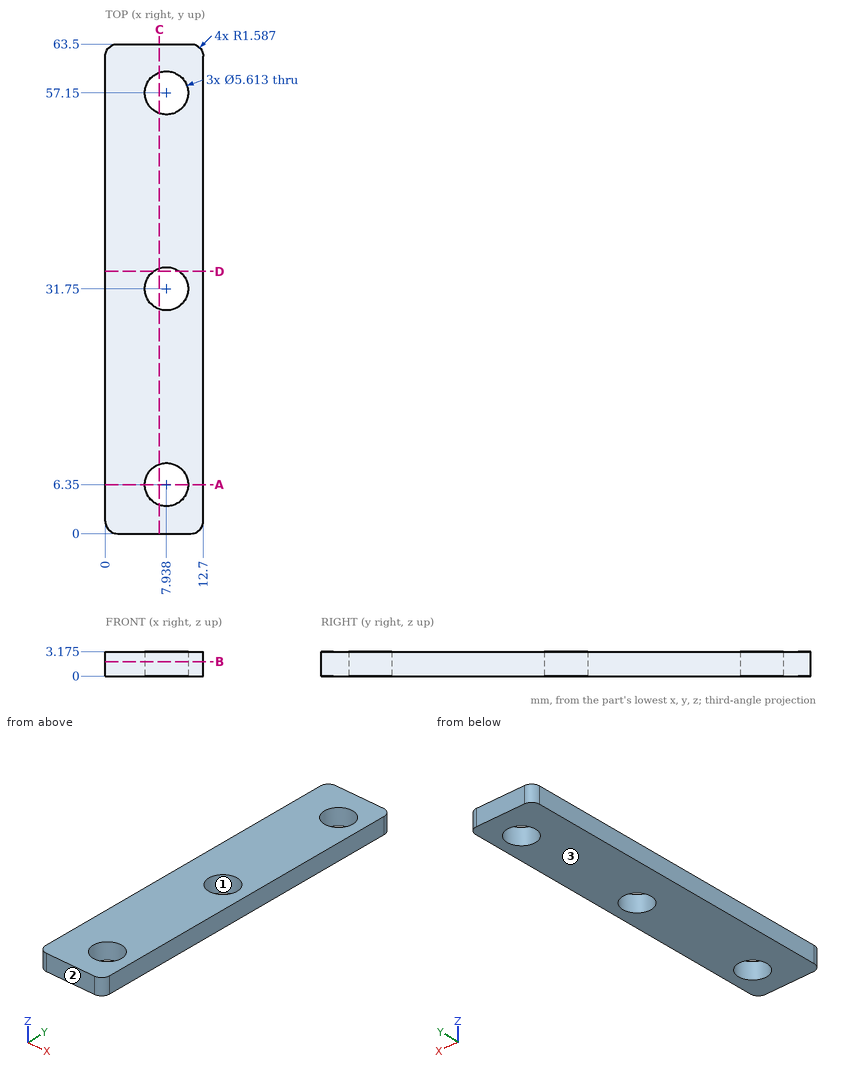
The drawing under review shows one solid part. Ordinate dimensions are in mm from its lowest x, y, z. Round coordinates to 2 decimals unless told otherwise and drop trailing zeros. Order: outer loops, then holes, each group sorted by start corner. A loop starts at its lowest first (then second) coordinate and runs counter-clockwise, first axis right, second up. Notation, with made-up numbers: (88.25, -22.5) - (125.25, -22.5) arc R21 cw to (125.25, -6.5) - close; hole circle Ø4 at (77.5, -4.5). An arc over 180 degrees is marked (long way). Return JSON: item names as keys, results as strings.
Q1. Consider section A-A on y = 6.35. Write out the cut boundary in (x, z) (1 decimal).
Computed values:
{"outline": "(0, 0) - (5.1, 0) - (5.1, 3.2) - (0, 3.2) - close; (10.7, 0) - (12.7, 0) - (12.7, 3.2) - (10.7, 3.2) - close"}
Q2. Consider section C-C on x = 7. Write out the cut boundary in (y, z) (1 decimal), plus the area to 3 significant figures.
Computed values:
{"outline": "(0, 0) - (3.7, 0) - (3.7, 3.2) - (0, 3.2) - close; (9, 0) - (29.1, 0) - (29.1, 3.2) - (9, 3.2) - close; (34.4, 0) - (54.5, 0) - (54.5, 3.2) - (34.4, 3.2) - close; (59.8, 0) - (63.5, 0) - (63.5, 3.2) - (59.8, 3.2) - close", "area": "151 mm2"}
Q3. Consider section B-B on z = 1.85. Give the number of separate pieces and of enclosed holes in the cut face, plus the area to 3 significant figures.
Computed values:
{"separate pieces": "1", "enclosed holes": "3", "area": "730 mm2"}
Q4. Consider section D-D on y = 34. Write out the cut boundary in (x, z) (1 decimal).
Computed values:
{"outline": "(0, 0) - (6.3, 0) - (6.3, 3.2) - (0, 3.2) - close; (9.6, 0) - (12.7, 0) - (12.7, 3.2) - (9.6, 3.2) - close"}
Q5. Wall thickness on L1, parallel to Y at x = 10.5, z = 2.4 (1 decimal); L2, parallel to Y at x = 7.5, z = 0.35; L3, parallel to Y at x = 0.75, z = 2.05: over which ranges is each line inside the solid? List them lowest first. Write a range as [from, to].
Computed values:
{"L1": "y = [0, 5.2], [7.5, 30.6], [32.9, 56], [58.3, 63.5]", "L2": "y = [0, 3.58], [9.12, 28.98], [34.52, 54.38], [59.92, 63.5]", "L3": "y = [0.24, 63.26]"}
Q6. The part is to be moulded in two halves that separate along Y. For the marked faces 1, 2 and 3, say which applies: pulls with the +Y half, pulls with the -Y half, needs draft (parallel to the pull), parting line crosses it, or undercut.
Computed values:
{"face 1": "undercut", "face 2": "pulls with the -Y half", "face 3": "needs draft"}
